Autodesk Inventor part; units mm, degrees
ref_plane "YZ Plane" through (0, 0, 0) normal (1, 0, 0) x (0, 1, 0)
ref_plane "XZ Plane" through (0, 0, 0) normal (0, 1, 0) x (-1, 0, 0)
ref_plane "XY Plane" through (0, 0, 0) normal (0, 0, 1) x (1, 0, 0)
sketch "Sketch1" plane through (0, 0, 0) normal (0, 1, 0) x (-1, 0, 0)
  arc A0 (1.5, -2.5981) -> (1.5, 2.5981) centre (3, 0) ccw
  arc A1 (-1.5, 2.5981) -> (-1.5, -2.5981) centre (-3, 0) ccw
  arc A2 (-1.5, 2.5981) -> (1.5, 2.5981) centre (0, 5.1962) ccw
  arc A3 (1.5, -2.5981) -> (-1.5, -2.5981) centre (0, -5.1962) ccw
  point P0 (0, 0)
  dimension "d0" = 6
  dimension "d1" = 6
  dimension "d2" = 6
  dimension "d3" = 3
  dimension "d4" = 6
  dimension "d5" = 6
extrude "Extrusion1" add sketch "Sketch1" along normal mid plane 5
sketch "Sketch2" plane through (0, 0, 0) normal (1, 0, 0) x (0, 1, 0)
  circle A0 centre (0, 0) radius 2
  dimension "d8" = 4
extrude "Extrusion2" add sketch "Sketch2" along normal blind 31
sketch "Sketch3" plane through (0, -2.5, 0) normal (0, -1, 0) x (1, 0, 0)
  arc A0 (-1.5, 2.5981) -> (-1.5, -2.5981) centre (-3, 0) ccw
  circle A1 centre (-3, 0) radius 1.5
  point P0 (0, 0)
  dimension "d11" = 3
extrude "Extrusion3" add sketch "Sketch3" along normal blind 3
hole "Hole1" at (3, -2.5, 0) direction (0, 1, 0) diameter 2.459 depth 8.8 tip angle 118
sketch "Sketch4" plane through (0, 0, 0) normal (0, 0, 1) x (1, 0, 0)
  line L0 (-1.5, -2.5) -> (-1.5, -5.5) construction
  line L1 (-1.5, -5.5) -> (-4.5, -5.5) construction
  line L2 (-4.5, -5.5) -> (-4.5, -2.5) construction
  line L3 (-4.5, -2.5) -> (-6, -2.5) construction
  line L4 (-6, -2.5) -> (-6, 2.5) construction
  line L5 (-6, 2.5) -> (1.7705, 2.5) construction
  line L6 (1.7705, 2.5) -> (1.7705, -2.5) construction
  line L7 (1.7705, -2.5) -> (-1.5, -2.5) construction
  line L8 (6, 2) -> (31, 2) construction
  line L9 (31, 2) -> (31, -2) construction
  line L10 (31, -2) -> (6, -2) construction
  line L11 (6, -2) -> (6, -2.5) construction
  line L12 (6, -2.5) -> (4.2295, -2.5) construction
  line L13 (4.2295, -2.5) -> (4.2295, 2.5) construction
  line L14 (4.2295, 2.5) -> (6, 2.5) construction
  line L15 (6, 2.5) -> (6, 2) construction
  circle A0 centre (29.5, 0) radius 0.55
  point P0 (0, 0)
  dimension "d23" = 1.1
  dimension "d24" = 1.5
extrude "Extrusion4" cut sketch "Sketch4" along normal mid plane 17.5
pattern_linear "Rectangular Pattern1" count 4 spacing 4 along (-1, 0, 0) of "Extrusion4"
chamfer "Chamfer1" distance 0.5 angle 45 1 edges at (31, -2, 0)
properties part number "500-178" material "ABS Plastic"
For this review, take the finished solid that the model builds, in its own axes (mm). A direction names the side the tool comes from. Round coordinates to 2 decimals unless told otherwise and drop trailing zeros. Write each loop counter-clockwise with the first axis right and the second up, starting at its lowest first coordinate (ties: lowest second). Pieces come first, ordered by that corner, then holes. Notation, with made-up numbers: M -36.75,22 L -26.75,22 A18 ccw -26.75,57 Z; hole C 85,78 d11. An arc over 180 degrees is marked long. One line per item, written item: value. Start each with the question number.
(1) We need section A-A (y = 0). Give the boundary of the cut face in (x, z).
(2) We need section D-D (x = 12). Give the boundary of the cut face in (y, z).
(3) The part is to be moulded in two halves that separate along X. For faces 3 (the cylindrical face through (-1.57, -3.98, -0.45)), 4 (the flat face through (0, -2.5, 0)), 5 (the cylindrical face through (1.78, 0.04, 0.16)), 6 (the cylindrical face through (18.025, 0.165, 0.028)), say which applies: released by +X, released by -X, zero draft, split by the parting line, or undercut.
(4) Insertion check: pin 1 (4 mm diameter, centred on x = 15, y = -2, fed in from -Z); pin 2 (1.4 mm diameter, centred on x = 29.5, y = 0, fed in from +Z); pin 3 (1.5 mm diameter, centred on x = 11.5, z = 1, fed in from +Y). Each pin has a flat end and moves straight along its axis. Give the tip position at first contact, or say it passes through.
(5) We need section B-B (z = 0). Give the boundary of the cut face in (x, y), and give its area (3 significant figures).
(6) Wall thickness on line 1 (X direction, y = 0, z = 0.9); line 2 (X direction, y = 0, z = -0.55); line 3 (Z direction, x = 3, y = 0.7): over which ranges is each line inside the solid? List them lowest first.
(7) Machinability: for faces 1 (the cylindrical face through (17.691, 1.847, 0.766)), 2 (the flat face through (-3, -5.5, 0)), which of the approach directions +Z, -Z, +X, -X, +Y, -Y give a long, thin tool a straight path to every point of the face, cutting with its end or side? Answer none if there is none.
(8) We need section C-C (x = 3). Give the boundary of the cut face in (y, z), and give its area (3 significant figures).
Result:
1. outline: M -1.5,-2.6 A3 cw 1.5,-2.6 A3 ccw 5.24,-2 L 16.95,-2 L 16.95,2 L 5.24,2 A3 ccw 1.5,2.6 A3 cw -1.5,2.6 A3 ccw long Z; M 18.05,-2 L 20.95,-2 L 20.95,2 L 18.05,2 Z; M 22.05,-2 L 24.95,-2 L 24.95,2 L 22.05,2 Z; M 26.05,-2 L 28.95,-2 L 28.95,2 L 26.05,2 Z; M 30.05,-2 L 30.5,-2 L 31,-1.5 L 31,1.5 L 30.5,2 L 30.05,2 Z; hole C 3,0 d2.46
2. outline: C 0,0 d4
3. face 3: split by the parting line
3. face 4: zero draft
3. face 5: undercut
3. face 6: undercut
4. pin 1: z = -2
4. pin 2: z = 2
4. pin 3: y = 1.98
5. outline: M -6,-2.5 L -4.5,-2.5 L -4.5,-5.5 L -1.5,-5.5 L -1.5,-2.5 L 1.77,-2.5 L 1.77,2.5 L -6,2.5 Z; M 4.23,-2.5 L 6,-2.5 L 6,-2 L 30.5,-2 L 31,-1.5 L 31,1.5 L 30.5,2 L 6,2 L 6,2.5 L 4.23,2.5 Z; hole C 17.5,0 d1.1; hole C 21.5,0 d1.1; hole C 25.5,0 d1.1; hole C 29.5,0 d1.1
5. area: 153 mm²
6. line 1: -5.86 to 2.16, 3.84 to 16.95, 18.05 to 20.95, 22.05 to 24.95, 26.05 to 28.95, 30.05 to 31
6. line 2: -5.95 to 1.9, 4.1 to 16.95, 18.05 to 20.95, 22.05 to 24.95, 26.05 to 28.95, 30.05 to 31
6. line 3: -3 to -1.23, 1.23 to 3
7. face 1: +X
7. face 2: +Z, -Z, +X, -X, -Y
8. outline: M -2.5,-3 L 2.5,-3 L 2.5,-1.23 L -2.5,-1.23 Z; M -2.5,1.23 L 2.5,1.23 L 2.5,3 L -2.5,3 Z
8. area: 17.7 mm²
